```python
from build123d import *

# Parameters (mm, degrees)
SKETCH1_W           = 25.4
SKETCH1_H           = 50.8
BOSS_EXTRUDE1_DEPTH = 6.096
CUT_EXTRUDE2_DEPTH  = 26.4
SKETCH4_W           = 15.24
SKETCH4_H           = 25.4
CUT_EXTRUDE3_DEPTH  = 7.096
SKETCH5_R           = 2.286
CUT_EXTRUDE4_DEPTH  = 2.54
CUT_EXTRUDE5_REACH  = 52.8
SKETCH6_R           = 0.9525


with BuildPart() as part:
    # Sketch1 → Boss-Extrude1 (new body)
    with BuildSketch(Plane(origin=(0, 0, 0), x_dir=(1, 0, 0), z_dir=(0, 1, 0))):
        Rectangle(SKETCH1_W, SKETCH1_H)
    extrude(amount=BOSS_EXTRUDE1_DEPTH)

    # Sketch3 → Cut-Extrude2 (cut, through all)
    with BuildSketch(Plane(origin=(12.7, 0, 0), x_dir=(0, 0, -1), z_dir=(1, 0, 0))):
        Polygon((-25.4, 6.096), (-25.4, 0), (-19.05, 0), align=None)
    extrude(amount=-CUT_EXTRUDE2_DEPTH, mode=Mode.SUBTRACT)

    # Sketch4 → Cut-Extrude3 (cut, through all)
    with BuildSketch(Plane.XZ):
        with Locations((0, -7.62)):
            Rectangle(SKETCH4_W, SKETCH4_H)
    extrude(amount=-CUT_EXTRUDE3_DEPTH, mode=Mode.SUBTRACT)

    # Sketch5 → Cut-Extrude4 (cut)
    with BuildSketch(Plane(origin=(0, 0, 5.08), x_dir=(-1, 0, 0), z_dir=(0, 0, -1))):
        with Locations((-3.81, 3.302)):
            Circle(SKETCH5_R)
        with Locations((3.81, 3.302)):
            Circle(SKETCH5_R)
    extrude(amount=-CUT_EXTRUDE4_DEPTH, mode=Mode.SUBTRACT)

    # Sketch6 → Cut-Extrude5 (cut, up to next)
    with BuildSketch(Plane(origin=(0, 0, -25.4), x_dir=(-1, 0, 0), z_dir=(0, 0, -1)), mode=Mode.PRIVATE) as cut_extrude5_sk1:
        with Locations((0, 3.048)):
            Circle(SKETCH6_R)
    cut_extrude5_tool1 = extrude(cut_extrude5_sk1.sketch, amount=-CUT_EXTRUDE5_REACH, mode=Mode.PRIVATE) & part.part
    add(cut_extrude5_tool1.solids().sort_by_distance((0, 3.048, -25.4))[0], mode=Mode.SUBTRACT)


solid = part.part
```
Geometry: final body of the model. Coordinates: model frame, mm. A direction names the side the tool comes from. Round coordinates to 2 decimals unless told otherwise and drop trailing zeros. Write each loop counter-clockwise with the first axis right and the second up, starting at its lowest first coordinate (ties: lowest second). Pieces come first, ordered by that corner, then holes. Notation, with made-up numbers: (-22, 6.25) -> (3, 6.25) arc R17 cw to (3, 24.25) -> close; hole circle Ø3 at (-13, 56). An arc over 180 degrees is marked (long way). Use CSV: the item, a comma, the result in double quotes. Start each with the question number.
Q1. Section B-B (z = -18). Return loops of the section in (x, y), plus the area to 3 significant figures.
Q2. Section D-D (y = 1.5). Return loops of the section in (x, z).
Q3. Pull-direction query (Z, two-part tool) for faces 4 (the face through (0.178, 3.005, 22.181)), 5 (the face through (0, 0, 6)), 6 (the face through (5.624, 1.911, 6.332)); classes: pulls with the +Z half, pulls with the -Z half, needs draft (parallel to the pull), parting line crosses it, or undercut.
Q4. First-contact query: pin 1 Ø1.5 at (x, y) = (0, 3.048) entering from -Z; pin 2 Ø1.8 at (x, y) = (-2.5, 3.5) entering from +Z. Flat tips, straight axial feed; report the tip coordinate or a pass-through.
Q5. Section C-C (x = -3.81). Return loops of the section in (y, z), plus the area to 3 significant figures.
Q6. Line query: L1, parallel to X at y = 5, z = -5.5; L2, parallel to Y at x = 0, z = -23.3; L3, parallel to Y at x = -3.81, z = 6.4. Output: solid intervals per line, ascending.
Q7. Section A-A (x = 0). Return loops of the section in (y, z), plus the area to 3 significant figures.
Q8. Reachability of faces 1 (the face through (0, 4, -23)), 2 (the face through (4, 3, 7.62)), 3 (the face through (0, 3, 5.08)) from +Z, -Z, +X, -X, +Y, -Y: full face, straight path, thin tool, end or side. Return the list, or none.
Result sheet:
1,outline,"(-12.7, 0) -> (-7.62, 0) -> (-7.62, 6.1) -> (-12.7, 6.1) -> close; (7.62, 0) -> (12.7, 0) -> (12.7, 6.1) -> (7.62, 6.1) -> close"
1,area,"61.9 mm²"
2,outline,"(-12.7, -25.4) -> (12.7, -25.4) -> (12.7, 20.61) -> (-12.7, 20.61) -> close; hole (-7.62, -20.32) -> (7.62, -20.32) -> (7.62, 5.08) -> (5.22, 5.08) -> (5.22, 7.62) -> (2.4, 7.62) -> (2.4, 5.08) -> (-2.4, 5.08) -> (-2.4, 7.62) -> (-5.22, 7.62) -> (-5.22, 5.08) -> (-7.62, 5.08) -> close"
3,face 4,"pulls with the +Z half"
3,face 5,"needs draft"
3,face 6,"undercut"
4,pin 1,"z = 5.08"
4,pin 2,"z = 23.63"
5,outline,"(0, -25.4) -> (6.1, -25.4) -> (6.1, -20.32) -> (0, -20.32) -> close; (0, 5.08) -> (1.02, 5.08) -> (1.02, 7.62) -> (5.59, 7.62) -> (5.59, 5.08) -> (6.1, 5.08) -> (6.1, 25.4) -> (0, 19.05) -> close"
5,area,"124 mm²"
6,L1,"-12.7 to -7.62, 7.62 to 12.7"
6,L2,"0 to 2.1, 4 to 6.1"
6,L3,"0 to 1.02, 5.59 to 6.1"
7,outline,"(0, -25.4) -> (2.1, -25.4) -> (2.1, -20.32) -> (0, -20.32) -> close; (0, 5.08) -> (6.1, 5.08) -> (6.1, 25.4) -> (0, 19.05) -> close; (4, -25.4) -> (6.1, -25.4) -> (6.1, -20.32) -> (4, -20.32) -> close"
7,area,"126 mm²"
8,face 1,"-Z"
8,face 2,"none"
8,face 3,"+Y, -Y"
